Can you work these out from the model? Positions are in its coordinate system, mm. Face numbers are marked on the shaded views. A direction names the side the tool comes from. Give positions to 0.01 mm unless a question says otherwise; leave off trailing zeros. Order: outer loops, then holes, each group sorted by start corner. A loop starts at its lowest first (then second) coordinate and runs counter-clockwise, first axis right, second up. Notation, with made-up numbers: M 30,84 L 78,84 A24 ccw 78,100 Z; hole C 54,29.5 d5. An arc over 180 degrees is marked long. Write each question's results on one line, items separated by ' | '.
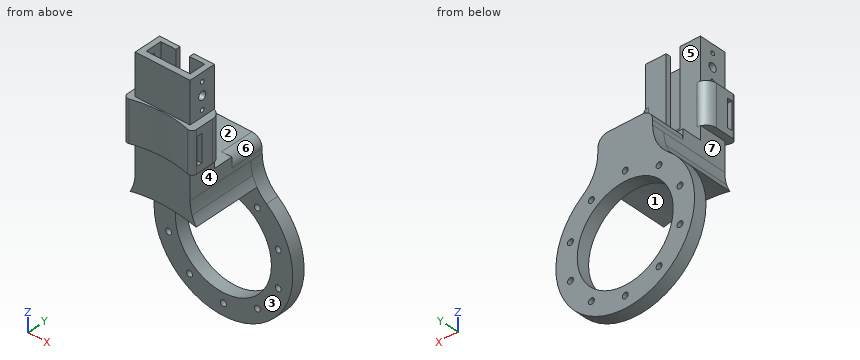
from build123d import *

# Parameters (mm, degrees)
SKETCH2_R           = 2.152402862
SKETCH2_R_2         = 35
BOSS_EXTRUDE2_DEPTH = 9.35
BOSS_EXTRUDE3_DEPTH = 50
CUT_EXTRUDE2_DEPTH  = 25
SKETCH8_W           = 40
SKETCH8_H           = 10
BOSS_EXTRUDE4_DEPTH = 20
BOSS_EXTRUDE5_DEPTH = 30
CUT_EXTRUDE4_DEPTH  = 56
SKETCH15_W          = 40
SKETCH15_H          = 20
BOSS_EXTRUDE6_DEPTH = 30
CUT_EXTRUDE5_DEPTH  = 55
SKETCH18_R          = 3
SKETCH18_R_2        = 1.5
CUT_EXTRUDE6_DEPTH  = 42


with BuildPart() as part:
    # Sketch2 → Boss-Extrude2 (new body)
    with BuildSketch(Plane(origin=(0, 0, 0), x_dir=(1, 0, 0), z_dir=(0, 1, 0))):
        with BuildLine():
            Line((-20, -74.081467259), (-20, -63.193139387))
            ThreePointArc((-20, -63.193139387), (-22.995916419, -50.124877454), (-31.385297997, -39.66671022))
            ThreePointArc((-31.385297997, -39.66671022), (0, 50.581467259), (31.385297997, -39.66671022))
            ThreePointArc((31.385297997, -39.66671022), (22.995916419, -50.124877454), (20, -63.193139387))
            Line((20, -63.193139387), (20, -74.081467259))
            Line((20, -74.081467259), (-20, -74.081467259))
        make_face()
        with Locations((0, 42)):
            Circle(SKETCH2_R, mode=Mode.SUBTRACT)
        with Locations((24.686980596, 33.978713764)):
            Circle(SKETCH2_R, mode=Mode.SUBTRACT)
        with Locations((39.944373684, 12.978713764)):
            Circle(SKETCH2_R, mode=Mode.SUBTRACT)
        with Locations((39.944373684, -12.978713764)):
            Circle(SKETCH2_R, mode=Mode.SUBTRACT)
        with Locations((24.686980596, -33.978713764)):
            Circle(SKETCH2_R, mode=Mode.SUBTRACT)
        with Locations((0, -42)):
            Circle(SKETCH2_R, mode=Mode.SUBTRACT)
        with Locations((-24.686980596, -33.978713764)):
            Circle(SKETCH2_R, mode=Mode.SUBTRACT)
        with Locations((-39.944373684, -12.978713764)):
            Circle(SKETCH2_R, mode=Mode.SUBTRACT)
        with Locations((-39.944373684, 12.978713764)):
            Circle(SKETCH2_R, mode=Mode.SUBTRACT)
        with Locations((-24.686980596, 33.978713764)):
            Circle(SKETCH2_R, mode=Mode.SUBTRACT)
        Circle(SKETCH2_R_2, mode=Mode.SUBTRACT)
    extrude(amount=BOSS_EXTRUDE2_DEPTH)

    # Sketch4 → Boss-Extrude3 (add)
    with BuildSketch(Plane.XZ):
        with BuildLine():
            Line((20, 74.081467259), (-20, 74.081467259))
            Line((-20, 74.081467259), (-20, 63.193139387))
            ThreePointArc((-20, 63.193139387), (-20.356412905, 58.582527267), (-21.417182941, 54.081467259))
            ThreePointArc((-21.417182941, 54.081467259), (-22.429520384, 51.366531516), (-23.699050675, 48.761920984))
            ThreePointArc((-23.699050675, 48.761920984), (0.438017323, 51.077240228), (24.422779297, 47.514944939))
            ThreePointArc((24.422779297, 47.514944939), (22.721671121, 50.70743662), (21.417182941, 54.081467259))
            ThreePointArc((21.417182941, 54.081467259), (20.356412905, 58.582527267), (20, 63.193139387))
            Line((20, 63.193139387), (20, 74.081467259))
        make_face()
    extrude(amount=BOSS_EXTRUDE3_DEPTH)

    # Sketch6 → Cut-Extrude2 (cut)
    with BuildSketch(Plane(origin=(0, 9.35, 0), x_dir=(1, 0, 0), z_dir=(0, 1, 0))):
        with BuildLine():
            Line((-12.5, -74.081467259), (-20, -74.081467259))
            Line((-20, -74.081467259), (-20, -66.581467259))
            ThreePointArc((-20, -66.581467259), (-17.803300859, -71.884768118), (-12.5, -74.081467259))
        make_face()
        with BuildLine():
            Line((12.5, -74.081467259), (20, -74.081467259))
            Line((20, -74.081467259), (20, -66.581467259))
            ThreePointArc((20, -66.581467259), (17.803300859, -71.884768118), (12.5, -74.081467259))
        make_face()
    extrude(amount=-CUT_EXTRUDE2_DEPTH, mode=Mode.SUBTRACT)

    # Sketch8 → Boss-Extrude4 (add)
    with BuildSketch(Plane(origin=(0, -50, 0), x_dir=(-1, 0, 0), z_dir=(0, -1, 0))):
        with Locations((0, -79.081467259)):
            Rectangle(SKETCH8_W, SKETCH8_H)
    extrude(amount=-BOSS_EXTRUDE4_DEPTH)

    # Sketch10 → Boss-Extrude5 (add)
    with BuildSketch(Plane.XY.offset(84.081467259)):
        with BuildLine():
            Line((-25, -37.5), (-25, -50.951484801))
            ThreePointArc((-25, -50.951484801), (-23.815635647, -53.339678092), (-21.197688536, -53.842210716))
            ThreePointArc((-21.197688536, -53.842210716), (0.197283847, -50.928235109), (21.59225623, -53.842210716))
            ThreePointArc((21.59225623, -53.842210716), (24.210203342, -53.339678092), (25.394567694, -50.951484801))
            Line((25.394567694, -50.951484801), (25.394567694, -37.5))
            ThreePointArc((25.394567694, -37.5), (23.197868553, -32.196699141), (17.894567694, -30))
            Line((17.894567694, -30), (-17.5, -30))
            ThreePointArc((-17.5, -30), (-22.803300859, -32.196699141), (-25, -37.5))
        make_face()
    extrude(amount=BOSS_EXTRUDE5_DEPTH)

    # Sketch11 → Cut-Extrude4 (cut)
    with BuildSketch(Plane.ZY.offset(25)):
        Polygon((109.081467259, -46.451484801), (109.081467259, -50.451484801), (99.081467259, -50.451484801), (89.081467259, -50.451484801), (89.081467259, -46.451484801), align=None)
    extrude(amount=-CUT_EXTRUDE4_DEPTH, mode=Mode.SUBTRACT)

    # Sketch15 → Boss-Extrude6 (add)
    with BuildSketch(Plane.XY.offset(114.081467259)):
        with Locations((0, -40)):
            Rectangle(SKETCH15_W, SKETCH15_H)
    extrude(amount=BOSS_EXTRUDE6_DEPTH)

    # Sketch17 → Cut-Extrude5 (cut)
    with BuildSketch(Plane.XY.offset(144.081467259)):
        Polygon((5, -30), (5, -33.451484801), (16, -33.451484801), (16, -45.451484801), (-16, -45.451484801), (-16, -33.451484801), (-5, -33.451484801), (-5, -30), align=None)
    extrude(amount=-CUT_EXTRUDE5_DEPTH, mode=Mode.SUBTRACT)

    # Sketch18 → Cut-Extrude6 (cut)
    with BuildSketch(Plane(origin=(20, 0, 0), x_dir=(0, 0, -1), z_dir=(1, 0, 0))):
        with Locations((-128.392898154, -40)):
            Circle(SKETCH18_R)
        with Locations((-118.892898154, -40)):
            Circle(SKETCH18_R_2)
        with Locations((-137.892898154, -40)):
            Circle(SKETCH18_R_2)
    extrude(amount=-CUT_EXTRUDE6_DEPTH, mode=Mode.SUBTRACT)


solid = part.part
(1) For the marked faces 5, 6 and 7, which set-ups out of +Z, -Z, +X, -X, +Y, -Y let a thin tool reach every point of the face, with its end or its side?
Data:
face 5: +Z, +X, -X, +Y | face 6: +Z, +X, +Y | face 7: -X, +Y, -Y
(2) I need wall thicknesses on L1, parallel to Y at x = -12.5, z = 132; L2, parallel to Z at x = 0, y = 3.25; L3, parallel to Y at x = -3, z = 100.5. Which ranges of each line are inside material? Lowest first, please. Write a range as from..to.
Data:
L1: y = -50..-45.45, -33.45..-30 | L2: z = -50.58..-44.15, -39.85..-35, 35..39.85, 44.15..74.08 | L3: y = -50.99..-50.45, -46.45..-45.45
(3) Imagine slicing it at A-A, the plane z = 0. Write out the boundary of the cut face in (x, y), plus the area to 3 significant figures.
Data:
outline: M -50.58,0 L -35,0 L -35,9.35 L -50.58,9.35 Z; M 35,0 L 50.58,0 L 50.58,9.35 L 35,9.35 Z | area: 291 mm2
(4) Imagine slicing it at D-D, the plane z = 42. Write out the boundary of the cut face in (x, y).
Data:
outline: M -28.77,0 L -2.15,0 L -2.15,9.35 L -28.77,9.35 Z; M 2.15,0 L 28.77,0 L 28.77,9.35 L 2.15,9.35 Z
(5) Imagine slicing it at B-B, the plane y = -7.5. Write out the boundary of the cut face in (x, z).
Data:
outline: M -23.7,48.76 A100 cw 24.42,47.51 A30 cw 20,63.19 L 20,66.58 A7.5 ccw 12.5,74.08 L -12.5,74.08 A7.5 ccw -20,66.58 L -20,63.19 A30 cw Z
(6) We'd pull the mould along Z, two halves only. Please class the marked faces 1, 2, 3 and 4: +Z half, -Z half, draft (parallel to the pull), parting line (faces both ways), or undercut.
Data:
face 1: -Z half | face 2: +Z half | face 3: draft | face 4: undercut
(7) Will these pins go through, and if not, where does the flat tip stop? P1, Ø16, axis at y = -37.5, z = 124.5, coming from the +X side; P2, Ø4, axis at x = -24.69, z = -33.98, coming from the -Y side; P3, Ø1.2, axis at x = -6.5, y = -47.5, coming from the -Z side; P4, Ø12, axis at x = -1.5, z = 100.5, coming from the +Y side.
Data:
P1: stops at x = 20 | P2: passes through | P3: stops at z = 50.99 | P4: stops at y = -30
(8) Imagine slicing it at C-C, the plane x = 0. Count the separate pieces of the cut face and the enclosed holes in it, plus the area to 3 significant figures.
Data:
separate pieces: 4 | enclosed holes: 1 | area: 2,080 mm2
